Here's how the part is built. I have some questions about the finished solid (model axes, mm). Face numbers are marked on the shaded views. A direction names the side the tool comes from. Coordinates: 2 decimals unless noted, no trailing zeros. Write each loop counter-clockwise with the first axis right and the second up, starting at its lowest first coordinate (ties: lowest second). Pieces come first, ordered by that corner, then holes. Notation, with made-up numbers: M 52.25,20 L 90.25,20 A26 ccw 90.25,57 Z; hole C 41,65.25 d5. An arc over 180 degrees is marked long. Use a Markdown table: item, result.
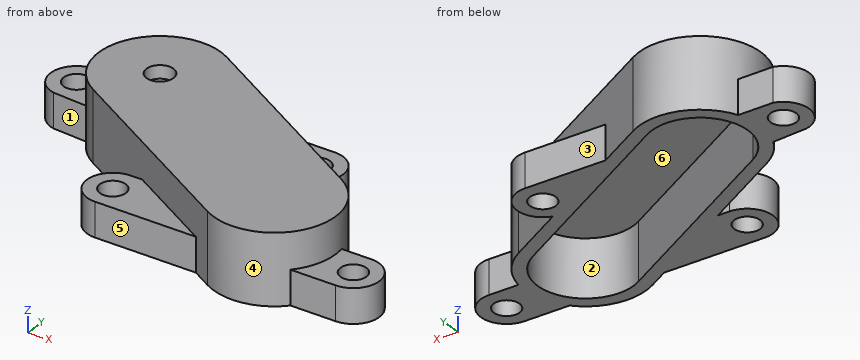
Autodesk Inventor part; units mm, degrees
ref_plane "YZ Plane" through (0, 0, 0) normal (1, 0, 0) x (0, 1, 0)
ref_plane "XZ Plane" through (0, 0, 0) normal (0, 1, 0) x (-1, 0, 0)
ref_plane "XY Plane" through (0, 0, 0) normal (0, 0, 1) x (1, 0, 0)
sketch "Sketch1" plane through (0, 0, 0) normal (0, 0, 1) x (1, 0, 0)
  line L0 (-103.0486, 32.008) -> (-29.0145, -10.8833) construction
  line L1 (-85.2832, 36.7398) -> (-33.7462, 6.8821)
  line L2 (-46.7799, -15.6151) -> (-98.3168, 14.2426)
  arc A0 (-85.2832, 36.7398) -> (-98.3168, 14.2426) centre (-91.8, 25.4912) ccw
  arc A1 (-46.7799, -15.6151) -> (-33.7462, 6.8821) centre (-40.2631, -4.3665) ccw
  circle A2 centre (-91.8, 25.4912) radius 4.5363 construction
  circle A3 centre (-43.5, -2.4912) radius 4.2314 construction
  line L3 (7.6716, 38.4912) -> (-163.6716, 38.4912) construction
  line L4 (-100.0713, 11.2141) -> (-48.5344, -18.6435)
  arc A4 (-48.5344, -18.6435) -> (-31.9917, 9.9106) centre (-40.2631, -4.3665) ccw
  line L5 (-31.9917, 9.9106) -> (-83.5287, 39.7682)
  arc A5 (-83.5287, 39.7682) -> (-100.0713, 11.2141) centre (-91.8, 25.4912) ccw
  point P0 (0, 0)
  point P1 (-66.0315, 10.5623)
  dimension "d0" = 3.5
extrude "Extrusion1" add sketch "Sketch1" along normal blind 15.5
sketch "Sketch2" plane through (0, 0, 15.5) normal (0, 0, 1) x (1, 0, 0)
  arc A0 (-83.5287, 39.7682) -> (-100.0713, 11.2141) centre (-91.8, 25.4912) ccw
  line L0 (-31.9917, 9.9106) -> (-83.5287, 39.7682)
  arc A1 (-48.5344, -18.6435) -> (-31.9917, 9.9106) centre (-40.2631, -4.3665) ccw
  line L1 (-100.0713, 11.2141) -> (-48.5344, -18.6435)
  point P0 (0, 0)
extrude "Extrusion2" add sketch "Sketch2" along normal blind 3.5
sketch "Sketch3" plane through (0, 0, 19) normal (0, 0, 1) x (1, 0, 0)
  circle A0 centre (-91.8, 25.4912) radius 2.5 construction
  circle A1 centre (-91.8, 25.4912) radius 3.65
  point P0 (0, 0)
  dimension "d5" = 7.3
extrude "Extrusion3" cut sketch "Sketch3" against normal through all
sketch "Sketch4" plane through (0, 0, 0) normal (0, 0, -1) x (-1, 0, 0)
  line L0 (121.4345, 25.6088) -> (42.3921, 25.6088) construction
  arc A0 (115.98, 18.7815) -> (116.2693, 32.3641) centre (114.4345, 25.6088) ccw
  arc A1 (49.3921, 32.6088) -> (49.3921, 18.6088) centre (49.3921, 25.6088) ccw
  circle A2 centre (114.4345, 25.6088) radius 3.5
  circle A3 centre (49.3921, 25.6088) radius 3.5
  line L1 (31.9917, 9.9106) -> (83.5287, 39.7682)
  line L2 (100.0713, 11.2141) -> (48.5344, -18.6435)
  arc A4 (100.0713, 11.2141) -> (83.5287, 39.7682) centre (91.8, 25.4912) ccw
  arc A5 (31.9917, 9.9106) -> (48.5344, -18.6435) centre (40.2631, -4.3665) ccw
  line L3 (116.2693, 32.3641) -> (106.8288, 32.3018)
  line L4 (115.98, 18.7815) -> (106.5624, 18.1208)
  line L5 (49.3921, 32.6088) -> (71.1708, 32.6088)
  line L6 (9.0132, -8.6068) -> (88.0556, -8.6068) construction
  line L7 (16.0132, -1.6068) -> (81.0556, -1.6068)
  line L8 (81.0556, -15.6068) -> (16.0132, -15.6068)
  arc A6 (16.0132, -1.6068) -> (16.0132, -15.6068) centre (16.0132, -8.6068) ccw
  arc A7 (81.0556, -15.6068) -> (81.0556, -1.6068) centre (81.0556, -8.6068) ccw
  circle A8 centre (16.0132, -8.6068) radius 3.5
  circle A9 centre (81.0556, -8.6068) radius 3.5
  point P0 (0, 0)
  point P1 (81.9133, 25.6088)
  point P2 (47.47, 18.8779)
  point P3 (48.5344, -8.6068)
  point P4 (77.9414, -1.6068)
  point P5 (53.7761, -15.6068)
  point P6 (28.1839, -15.6068)
  point P7 (23.9955, -1.6068)
  dimension "d8" = 7
  dimension "d9" = 7
  dimension "d12" = 65.0425
  dimension "d13" = 65.0425
  dimension "d14" = 7
  dimension "d15" = 7
  dimension "d16" = 7
  dimension "d17" = 7
  dimension "d18" = 7
extrude "Extrusion4" add sketch "Sketch4" against normal blind 9.25 contours L4 A4 L3 A0 | L7 A7 L8 L2 | L1 A1 L5 | A5 L8 A6 L7
equation "\"d13\" = d12"
equation "\"d14\" = d15"
equation "\"d16\" = d15"
properties part number "Y belt Cover"
1. We'd pull the mould along Y, two halves only. Please class the marked faces 1, 2 and 3: +Y half, -Y half, draft (parallel to the pull), parting line (faces both ways), or undercut.
Answers follow:
| item | result |
|---|---|
| face 1 | -Y half |
| face 2 | undercut |
| face 3 | +Y half |
2. Suppose I cut it at C-C on x = -91.8. Write out the boundary of the cut face in (y, z).
Answers follow:
| item | result |
|---|---|
| outline | M 6.42,0 L 10.47,0 L 10.47,15.5 L 21.84,15.5 L 21.84,19 L 6.42,19 Z; M 29.14,15.5 L 38.49,15.5 L 38.49,0 L 41.99,0 L 41.99,19 L 29.14,19 Z |
3. Suppose I cut it at B-B on y = -3. Write out the boundary of the cut face in (x, z).
Answers follow:
| item | result |
|---|---|
| outline | M -85.25,0 L -68.55,0 L -68.55,15.5 L -27.34,15.5 L -27.34,0 L -11.82,0 L -11.82,9.25 L -23.82,9.25 L -23.82,19 L -75.54,19 L -75.54,9.25 L -85.25,9.25 Z |
4. I need wall thicknesses on probe 1 along X at (y, z) = (-9, 8.75); probe 2 along X at (y, z) = (37, 1.5); probe 3 along Z at (x, y) = (-48, 3). Which ranges of each line are inside material? Lowest first, please.
Answers follow:
| item | result |
|---|---|
| probe 1 | x = -88.04 to -84.53, -77.58 to -58.2, -28.12 to -19.49, -12.54 to -9.02 |
| probe 2 | x = -103.62 to -97.85, -85.75 to -78.75 |
| probe 3 | z = 15.5 to 19 |
5. Suppose I cut it at D-D on y = 34. Write out the boundary of the cut face in (x, z), and give its area (3 significant figures).
Answers follow:
| item | result |
|---|---|
| outline | M -105.94,0 L -101.63,0 L -101.63,15.5 L -80.55,15.5 L -80.55,0 L -73.57,0 L -73.57,19 L -105.94,19 Z |
| area | 288 mm2 |
6. Which directions (+Z, -Z, +X, -X, +Y, -Y) give clear straight access to the entire face, cutting with the end or side of a thin tool? Please do the marked faces 4, 5 and 6.
Answers follow:
| item | result |
|---|---|
| face 4 | +Z |
| face 5 | +Z, -Z, -X, -Y |
| face 6 | -Z |
7. Will these pins go through, and if not, where does the flat tip stop? pin 1 Ø10 at (x, z) = (-21, 3.5) entering from -Y; pin 2 Ø5.5 at (x, y) = (-49.39, 25.61) entering from +Z; pin 3 Ø6.5 at (x, z) = (-20.5, 3) entering from +Y; pin 4 Ø0.9 at (x, z) = (-79, 3) entering from +Y.
Answers follow:
| item | result |
|---|---|
| pin 1 | stops at y = -15.61 |
| pin 2 | passes through |
| pin 3 | stops at y = -1.61 |
| pin 4 | stops at y = 37.41 |
